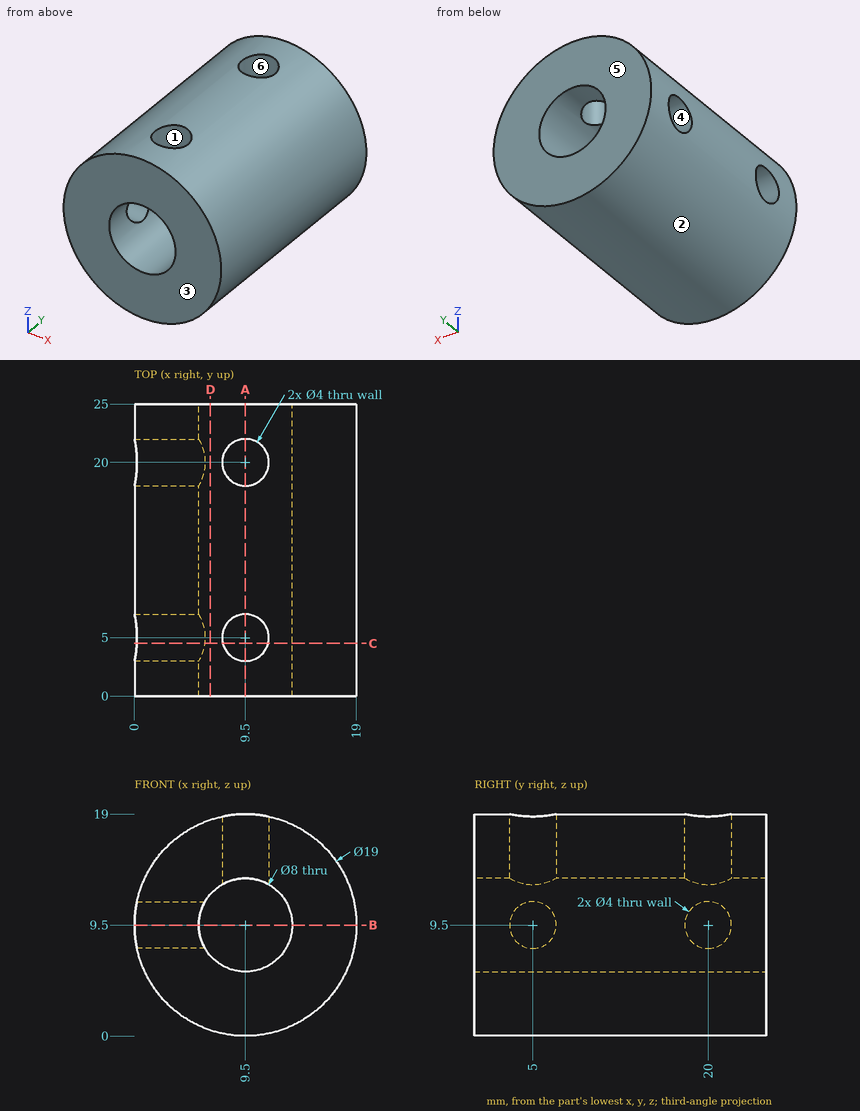
Part print with two shaded views. Sizes in mm from the minimum x, y, z corner. A direction names the side the tool comes from. Coordinates: 2 decimals unless noted, no trailing zeros. Order: outer loops, then holes, each group sorted by start corner. A loop starts at its lowest first (then second) coordinate and runs counter-clockwise, first axis right, second up. Notation, with made-up numbers: (40, 56.25) - (46, 56.25) arc R25 ccw to (46, 88.25) - close; hole circle Ø1 at (55, 8). An arc over 180 degrees is marked (long way). Write item = value, one per line. Start each with the question number.
1) 3-axis set-ups, long thin cutter, end or side, ignore diameter. For the marked faces 4, 5 and 6: which of +Z, -Z, +X, -X, +Y, -Y reach the whole face in a straight line?
2) Flat gauge pins, fed straight in: pin 1 Ø3 at (y, z) = (10, 6) entering from -X; pin 2 Ø6 at (x, y) = (4, 4) entering from +Z. Where does each tip first touch, or does it go through?
3) Saw through at A-A on x = 9.5. Write the cut outline in (y, z).
4) Saw through at C-C on y = 4.5. Write the cut outline in (x, z), then the cut area to 3 significant figures.
5) Saw through at D-D on x = 6.5. Write the cut outline in (y, z), then the cut area to 3 significant figures.
6) Saw through at B-B on z = 9.5. Write the cut outline in (x, y).
7) Wall check: line 1 along Y through (x, z) = (10.5, 17.75); line 2 along X through (y, z) = (6, 15.75); line 3 along Z through (x, y) = (13, 12.25). Give the ranges that are in metal, low to high. Write a range as from..to.
8) Two-plate mould, pull along X, no slides. Class the marked faces 1, 2 and 3: pulls with the +X half, pulls with the -X half, needs draft (parallel to the pull), parting line crosses it, or undercut.
From the geometry:
q1.face_4 = -X
q1.face_5 = +Z, -Z, +X, -X, +Y
q1.face_6 = +Z
q2.pin_1 = 0.21
q2.pin_2 = 18.67
q3.outline = (0, 0) - (25, 0) - (25, 5.5) - (0, 5.5) - close; (0, 13.5) - (3, 13.5) - (3, 19) - (0, 19) - close; (7, 13.5) - (18, 13.5) - (18, 19) - (7, 19) - close; (22, 13.5) - (25, 13.5) - (25, 19) - (22, 19) - close
q4.outline = (0.2, 7.56) arc R9.5 ccw (long way) to (11.44, 18.8) - (11.44, 13) arc R4 cw (long way) to (6, 7.56) - close; (0.2, 11.44) - (6, 11.44) arc R4 cw to (7.56, 13) - (7.56, 18.8) arc R9.5 ccw to start
q4.area = 190 mm^2
q5.outline = (0, 0.49) - (25, 0.49) - (25, 6.85) - (0, 6.85) - close; (0, 12.15) - (25, 12.15) - (25, 18.51) - (0, 18.51) - close
q5.area = 318 mm^2
q6.outline = (0, 0) - (5.5, 0) - (5.5, 3) - (0, 3) - close; (0, 7) - (5.5, 7) - (5.5, 18) - (0, 18) - close; (0, 22) - (5.5, 22) - (5.5, 25) - (0, 25) - close; (13.5, 0) - (19, 0) - (19, 25) - (13.5, 25) - close
q7.line_1 = 0..3.27, 6.73..18.27, 21.73..25
q7.line_2 = 2.35..7.77, 11.23..16.65
q7.line_3 = 0.67..7.56, 11.44..18.33
q8.face_1 = undercut
q8.face_2 = parting line crosses it
q8.face_3 = needs draft
